Input: part model. Units: mm. Frame: model coordinates. Face numbers are marked on the shaded views. Give positions to 0.01 mm unless a question says otherwise; leave off trailing zeros. Loops run counter-clockwise (first coordinate to the right, second up) from the corner with the lowest first, then second, coordinate; pieces in that order, holes last. Notation, with made-up numbers: M -14,52 L 13,52 A26 ccw 13,84 Z; hole C 70.25,15 d3. An arc over 180 degrees is marked long. Use CSV: the item, a comma, the result in double quotes. Start each with the question number.
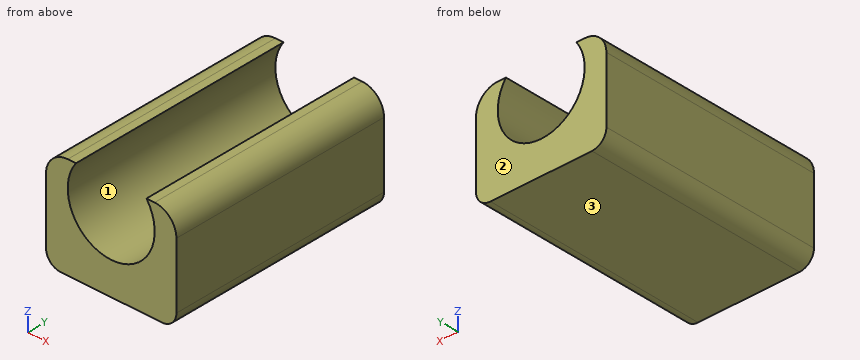
from build123d import *

# Parameters (mm, degrees)
SKETCH_W     = 18
SKETCH_H     = 14
PAD_DEPTH    = 15.5
FILLET_R     = 2
SKETCH001_R  = 6
POCKET_DEPTH = 31.001
FILLET001_R  = 3


with BuildPart() as part:
    # Sketch → Pad (new body, symmetric)
    with BuildSketch(Plane.XZ):
        Rectangle(SKETCH_W, SKETCH_H)
    extrude(amount=PAD_DEPTH, both=True)

    # Fillet
    fillet_edges = [part.edges().sort_by_distance(p)[0] for p in [
        (-9, 0, -7),
        (9, 0, -7),
    ]]
    fillet(fillet_edges, radius=FILLET_R)

    # Sketch001 → Pocket (cut, through all)
    with BuildSketch(Plane.XZ.offset(15.5)):
        with Locations((0, 3.5)):
            Circle(SKETCH001_R)
    extrude(amount=-POCKET_DEPTH, mode=Mode.SUBTRACT)

    # Fillet001
    fillet001_edges = [part.edges().sort_by_distance(p)[0] for p in [
        (9, 0, 7),
        (-9, 0, 7),
    ]]
    fillet(fillet001_edges, radius=FILLET001_R)


solid = part.part
Item 1: Section C-C (x = 0). Output: boundary loops of the cut face in (y, z).
Item 2: Section A-A (z = 3.5). Output: boundary loops of the cut face in (x, y).
Item 3: First-contact query: pin 1 Ø2 at (x, y) = (3.5, -1) entering from +Z. Flat tip, straight axial feed; report the tip coordinate or a pass-through.
Item 4: Material intervals for line 1 (X direction, y = -7, z = 3.5); line 2 (Z direction, x = 0, y = 3); line 3 (X direction, y = 4, z = -1.5), sorted ascending.
Item 5: Section D-D (z = -1.25). Output: boundary loops of the cut face in (x, y), then the cut area to 3 significant figures.
Item 6: Mould query, pull axis Z, two halves, no side actions, for the marked faces 1, 2 and 3. Classes: +Z half, -Z half, draft (parallel to the pull), parting line (faces both ways), or undercut.
Item 7: Section B-B (y = 13). Output: boundary loops of the cut face in (x, z).
Recorded:
1,outline,"M -15.5,-7 L 15.5,-7 L 15.5,-2.5 L -15.5,-2.5 Z"
2,outline,"M -9,-15.5 L -6,-15.5 L -6,15.5 L -9,15.5 Z; M 6,-15.5 L 9,-15.5 L 9,15.5 L 6,15.5 Z"
3,pin 1,"z = -0.47"
4,line 1,"-9 to -6, 6 to 9"
4,line 2,"-7 to -2.5"
4,line 3,"-9 to -3.32, 3.32 to 9"
5,outline,"M -9,-15.5 L -3.67,-15.5 L -3.67,15.5 L -9,15.5 Z; M 3.67,-15.5 L 9,-15.5 L 9,15.5 L 3.67,15.5 Z"
5,area,"331 mm²"
6,face 1,"undercut"
6,face 2,"draft"
6,face 3,"-Z half"
7,outline,"M -9,-5 A2 ccw -7,-7 L 7,-7 A2 ccw 9,-5 L 9,4 A3 ccw 6,7 L 4.87,7 A6 cw long -4.87,7 L -6,7 A3 ccw -9,4 Z"
